```python
from build123d import *

# Parameters (mm, degrees)
F0_W     = 119.197724
F0_H     = 66.822962
F1_DEPTH = 12.7
F2_W     = 93.797724
F2_H     = 66.037954
F3_DEPTH = 50.8
F4_R     = 21.859631
F5_DEPTH = 123.444
F6_W     = 78.557724
F6_H     = 17.734622
F7_DEPTH = 38.1


with BuildPart() as f1:
    # F0 (on Top) → F1 (new body)
    with BuildSketch(Plane.XY):
        Rectangle(F0_W, F0_H)
    extrude(amount=F1_DEPTH)

    # F2 (on Top) → F3 (join)
    with BuildSketch(Plane.XY):
        Rectangle(F2_W, F2_H)
    extrude(amount=F3_DEPTH)

    # F4 (on Top) → F5 (cut)
    with BuildSketch(Plane.XY):
        with Locations((0, 34.088746)):
            Circle(F4_R)
    extrude(amount=F5_DEPTH, mode=Mode.SUBTRACT)

    # F6 (on face) → F7 (cut)
    with BuildSketch(Plane.XY.offset(50.8)):
        with Locations((0, -24.107311)):
            Rectangle(F6_W, F6_H)
    extrude(amount=-F7_DEPTH, mode=Mode.SUBTRACT)


solid = f1.part
```
Design review of the part built by this model. Coordinates are the model's own, in mm. A direction names the side the tool comes from. Coordinates: 2 decimals unless noted, no trailing zeros. Loops run counter-clockwise (first coordinate to the right, second up) from the corner with the lowest first, then second, coordinate; pieces in that order, holes last. Notation, with made-up numbers: (-5.5, -35.5) - (23.5, -35.5) arc R21 ccw to (23.5, -28.5) - close; hole circle Ø1 at (-11.75, 30.5). An arc over 180 degrees is marked (long way). Use CSV: the item, a comma, the result in double quotes. Start each with the question number.
1) The part is to be moulded in two halves that separate along Y. For faces 1 (the flat face through (-41, 33.411, 6)), 2 (the flat face through (-1, -15.24, 32)), 3 (the flat face through (-46.899, 0, 31)), say which applies: +Y half, -Y half, draft (parallel to the pull), parting line (faces both ways), or undercut.
2) Tool access review of faces 4 (the flat face through (-59.599, 0, 6)), 5 (the flat face through (59.599, 0, 6)), 6 (the flat face through (-35, 33.019, 31)), 7 (the flat face through (46.899, 0, 31)), 8 (the flat face through (39.279, -24, 32)): name each direction out of +Z, -Z, +X, -X, +Y, -Y from which nothing blocks a thin tool from reaching the whole face with its end or side.
3) Consider section B-B on y = 21.5. Write out the cut boundary in (x, z), then the cut area to 3 significant figures.
4) Consider section A-A on z = 21.5. Write out the cut boundary in (x, y), then the cut area to 3 significant figures.
5) Wall thickness on L1, parallel to X at y = -20.5, z = 32.5; L2, parallel to Z at x = 8, y = -23.5; L3, parallel to X at y = 8, z = 13: over which ranges is each line inside the solid? List them lowest first. Write a range as from..to.
6) Consider section D-D on y = 1. Write out the cut boundary in (x, z).
7) Consider section C-C on x = 0. Write out the cut boundary in (y, z).
8) For pin 1 Ø6 at (y, z) = (-5.5, 33.5) entering from +X; pin 2 Ø1.5 at (x, z) = (43.5, 40.5) entering from +Y; pin 3 Ø11.5 at (x, z) = (2, 27) entering from -Y, all flat-tipped, find the tip position at first contact; note any pin that passes through.
Geometry says:
1,face 1,"+Y half"
1,face 2,"undercut"
1,face 3,"draft"
2,face 4,"+Z, -Z, -X, +Y, -Y"
2,face 5,"+Z, -Z, +X, +Y, -Y"
2,face 6,"+Z, +X, -X, +Y"
2,face 7,"+Z, +X, +Y, -Y"
2,face 8,"+Z"
3,outline,"(-59.6, 0) - (-17.87, 0) - (-17.87, 50.8) - (-46.9, 50.8) - (-46.9, 12.7) - (-59.6, 12.7) - close; (17.87, 0) - (59.6, 0) - (59.6, 12.7) - (46.9, 12.7) - (46.9, 50.8) - (17.87, 50.8) - close"
3,area,"3,270 mm^2"
4,outline,"(-46.9, -33.02) - (46.9, -33.02) - (46.9, 33.02) - (21.83, 33.02) arc R21.86 cw to (-21.83, 33.02) - (-46.9, 33.02) - close; hole (-39.28, -32.97) - (39.28, -32.97) - (39.28, -15.24) - (-39.28, -15.24) - close"
4,area,"4,100 mm^2"
5,L1,"-46.9..-39.28, 39.28..46.9"
5,L2,"0..12.7"
5,L3,"-46.9..46.9"
6,outline,"(-59.6, 0) - (59.6, 0) - (59.6, 12.7) - (46.9, 12.7) - (46.9, 50.8) - (-46.9, 50.8) - (-46.9, 12.7) - (-59.6, 12.7) - close"
7,outline,"(-33.41, 0) - (12.23, 0) - (12.23, 50.8) - (-15.24, 50.8) - (-15.24, 12.7) - (-32.97, 12.7) - (-32.97, 50.8) - (-33.02, 50.8) - (-33.02, 12.7) - (-33.41, 12.7) - close"
8,pin 1,"x = 46.9"
8,pin 2,"y = 33.02"
8,pin 3,"y = -33.02"
